```python
from build123d import *

# Parameters (mm, degrees)
SKETCH1_W           = 20
SKETCH1_H           = 27
BOSS_EXTRUDE1_DEPTH = 1
SKETCH2_W           = 8
SKETCH2_H           = 8
BOSS_EXTRUDE2_DEPTH = 2
SKETCH2_3_R         = 4
BOSS_EXTRUDE3_DEPTH = 7
SKETCH3_W           = 10
SKETCH3_H           = 4
SKETCH3_W_2         = 9.6
SKETCH3_H_2         = 3.6
EXTRUDE_THIN1_DEPTH = 6


with BuildPart() as part:
    # Sketch1 → Boss-Extrude1 (new body)
    with BuildSketch(Plane.XY):
        Rectangle(SKETCH1_W, SKETCH1_H)
    extrude(amount=BOSS_EXTRUDE1_DEPTH)

    # Sketch2 → Boss-Extrude2 (add)
    with BuildSketch(Plane(origin=(0, 0, 0), x_dir=(-1, 0, 0), z_dir=(0, 0, -1))):
        with Locations((0, 6.5)):
            Rectangle(SKETCH2_W, SKETCH2_H)
    extrude(amount=BOSS_EXTRUDE2_DEPTH)

    # Sketch2<3> → Boss-Extrude3 (add)
    with BuildSketch(Plane(origin=(0, 0, 0), x_dir=(-1, 0, 0), z_dir=(0, 0, -1))):
        with Locations((0, 6.5)):
            Circle(SKETCH2_3_R)
    extrude(amount=BOSS_EXTRUDE3_DEPTH)

    # Sketch3 → Extrude-Thin1 (add)
    with BuildSketch(Plane.XY.offset(1)):
        with Locations((0, -11.5)):
            Rectangle(SKETCH3_W, SKETCH3_H)
        with Locations((0, -11.5)):
            Rectangle(SKETCH3_W_2, SKETCH3_H_2, mode=Mode.SUBTRACT)
    extrude(amount=EXTRUDE_THIN1_DEPTH)


solid = part.part
```
Read the model definition and answer for the solid it produces. Units are mm, in the model's axes. A direction names the side the tool comes from. Give positions to 0.01 mm unless a question says otherwise; leave off trailing zeros. Order: outer loops, then holes, each group sorted by start corner. A loop starts at its lowest first (then second) coordinate and runs counter-clockwise, first axis right, second up. Notation, with made-up numbers: (-34, -18) -> (-3, -18) arc R17 cw to (-3, -11) -> close; hole circle Ø9 at (-15.5, 20). An arc over 180 degrees is marked (long way). One line per item, written item: value. Start each with the question number.
(1) A tool of negligible diameter and unlimited length cuts with its end or side. For faces 1 (the flat face through (4, 6, -1)), 2 (the flat face through (0, -9.5, 4)), 3 (the flat face through (0, 10.5, -1)), 4 (the flat face through (3, 10, -2)), from which of +Z, -Z, +X, -X, +Y, -Y can it reach the whole face along a straight path? Write none if from no direction.
(2) The part is cut by section C-C (x = 7.25). Determine the outline of the cut face in (y, z), and give its area (3 significant figures).
(3) For a pull along Y with two mould halves and no side action, classify faces 5 (the flat face through (0, -13.5, 3)), 6 (the flat face through (4.8, -12, 4)), 7 (the flat face through (0, 0, 1)) as released by +Y, released by -Y, zero draft, split by the parting line, or undercut.
(4) The part is cut by section B-B (y = -12). Determine the outline of the cut face in (x, z), and give its area (3 significant figures).
(5) The part is cut by section D-D (y = -1.5). Determine the outline of the cut face in (x, z), and give its area (3 significant figures).
(6) Flat-ended cylindrical pins translate along their axes: P1, Ø1, axis at y = 8.5, z = -3.5, coming from the +X side; P2, Ø6, axis at x = 2.5, y = -6.5, coming from the -Z side; P3, Ø6, axis at x = -7, z = 2.5, coming from the +Y side; P4, Ø3, axis at y = 6, z = -5, coming from the -X side. Find the tip coordinate at first contact, or state that the pin passes through.
(7) The part is cut by section A-A (z = 3). Determine the outline of the cut face in (x, y), and give its area (3 significant figures).
(8) Straight lines are drawn through the part: L1, parallel to Y at x = -4.25, z = 2; L2, parallel to Z at x = 2.75, y = 1.25; L3, parallel to Z at x = -2.5, y = 8.75. For each, find the intervals that lie inside material, in ascending order.
Taken from the geometry:
1. face 1: -Z, +X, +Y, -Y
1. face 2: +Z, +X, -X, +Y
1. face 3: -Z, +X, -X, +Y
1. face 4: -Z, +X, +Y
2. outline: (-13.5, 0) -> (13.5, 0) -> (13.5, 1) -> (-13.5, 1) -> close
2. area: 27.0 mm^2
3. face 5: released by -Y
3. face 6: undercut
3. face 7: zero draft
4. outline: (-10, 0) -> (10, 0) -> (10, 1) -> (5, 1) -> (5, 7) -> (4.8, 7) -> (4.8, 1) -> (-4.8, 1) -> (-4.8, 7) -> (-5, 7) -> (-5, 1) -> (-10, 1) -> close
4. area: 22.4 mm^2
5. outline: (-10, 0) -> (10, 0) -> (10, 1) -> (-10, 1) -> close
5. area: 20.0 mm^2
6. P1: x = 3.71
6. P2: z = 0
6. P3: y = 13.5
6. P4: x = -4
7. outline: (-5, -13.5) -> (5, -13.5) -> (5, -9.5) -> (-5, -9.5) -> close; hole (-4.8, -13.3) -> (4.8, -13.3) -> (4.8, -9.7) -> (-4.8, -9.7) -> close
7. area: 5.44 mm^2
8. L1: -13.5 to -13.3, -9.7 to -9.5
8. L2: 0 to 1
8. L3: -7 to 1
